Part model, mm, in its own coordinate system. Round coordinates to 2 decimals unless told otherwise and drop trailing zeros. Write each loop counter-clockwise with the first axis right and the second up, starting at its lowest first coordinate (ties: lowest second). Pieces come first, ordered by that corner, then holes.
1) Saw through at B-B on x = 0. Write the cut outline in (y, z), and give its area (3 significant figures).
2) Drill centre lines: L1, parallel to X at y = 1.85, z = 24.5; L2, parallel to X at y = 2.3, z = -8; L3, parallel to X at y = 1.8, z = -25.5. Where is each one in solid material? Low to high.
3) Saw through at A-A on z = 3.5. Write the cut outline in (x, y).
4) Saw through at C-C on y = 1.35. Count the separate pieces of the cut face and the enclosed holes in it, and give its area (3 significant figures).
5) Saw through at D-D on x = -42. Write the cut outline in (y, z).
6) Flat gauge pin, fed straight in: pin 1 (2.5 mm diameter, centred on x = -55, z = -24.5, fed in from +Y). Where does the tip first touch, or does it go through?
```python
from build123d import *

# Parameters (mm, degrees)
SKETCH_1_W          = 120
SKETCH_1_H          = 60
EXTRUDE_1_DEPTH     = 3
SKETCH_2_R          = 1.5
CUT_EXTRUDE_1_DEPTH = 68.149087857
SKETCH_3_R          = 1.5
CUT_EXTRUDE_2_DEPTH = 68.149087857
FILLET_1_R          = 5
SKETCH_4_W          = 30
SKETCH_4_H          = 40
CUT_EXTRUDE_3_DEPTH = 68.149087857
FILLET_2_R          = 5


with BuildPart() as part:
    # Sketch 1 → Extrude 1 (new body)
    with BuildSketch(Plane(origin=(0, 0, 0), x_dir=(1, 0, 0), z_dir=(0, 1, 0))):
        Rectangle(SKETCH_1_W, SKETCH_1_H)
    extrude(amount=EXTRUDE_1_DEPTH)

    # Sketch 2 → Cut-Extrude 1 (cut, through all)
    with BuildSketch(Plane(origin=(0, 3, 0), x_dir=(1, 0, 0), z_dir=(0, 1, 0))):
        with Locations(Location((-55, 24.5, 0), (0, 0, 270))):
            Circle(SKETCH_2_R)
        with Locations(Location((-15, 24.5, 0), (0, 0, 270))):
            Circle(SKETCH_2_R)
        with Locations(Location((-55, -24.5, 0), (0, 0, 90))):
            Circle(SKETCH_2_R)
        with Locations(Location((-15, -24.5, 0), (0, 0, 90))):
            Circle(SKETCH_2_R)
        with Locations(Location((15, -24.5, 0), (0, 0, 270))):
            Circle(SKETCH_2_R)
        with Locations(Location((55, -24.5, 0), (0, 0, 270))):
            Circle(SKETCH_2_R)
        with Locations(Location((15, 24.5, 0), (0, 0, 90))):
            Circle(SKETCH_2_R)
        with Locations(Location((55, 24.5, 0), (0, 0, 90))):
            Circle(SKETCH_2_R)
    extrude(amount=-CUT_EXTRUDE_1_DEPTH, mode=Mode.SUBTRACT)

    # Sketch 3 → Cut-Extrude 2 (cut, through all)
    with BuildSketch(Plane(origin=(0, 3, 0), x_dir=(1, 0, 0), z_dir=(0, 1, 0))):
        with Locations(Location((0, 15, 0), (0, 0, 270))):
            Circle(SKETCH_3_R)
        with Locations(Location((0, -15, 0), (0, 0, 90))):
            Circle(SKETCH_3_R)
    extrude(amount=-CUT_EXTRUDE_2_DEPTH, mode=Mode.SUBTRACT)

    # Fillet 1
    fillet_1_edges = [part.edges().sort_by_distance(p)[0] for p in [
        (60, 1.5, 30),
        (-60, 1.5, 30),
        (-60, 1.5, -30),
        (60, 1.5, -30),
    ]]
    fillet(fillet_1_edges, radius=FILLET_1_R)

    # Sketch 4 → Cut-Extrude 3 (cut, through all)
    with BuildSketch(Plane(origin=(0, 3, 0), x_dir=(1, 0, 0), z_dir=(0, 1, 0))):
        with Locations((35, 0)):
            Rectangle(SKETCH_4_W, SKETCH_4_H)
        with Locations((-35, 0)):
            Rectangle(SKETCH_4_W, SKETCH_4_H)
    extrude(amount=-CUT_EXTRUDE_3_DEPTH, mode=Mode.SUBTRACT)

    # Fillet 2
    fillet_2_edges = [part.edges().sort_by_distance(p)[0] for p in [
        (50, 1.5, -20),
        (50, 1.5, 20),
        (20, 1.5, 20),
        (20, 1.5, -20),
        (-20, 1.5, -20),
        (-20, 1.5, 20),
        (-50, 1.5, 20),
        (-50, 1.5, -20),
    ]]
    fillet(fillet_2_edges, radius=FILLET_2_R)


solid = part.part
```
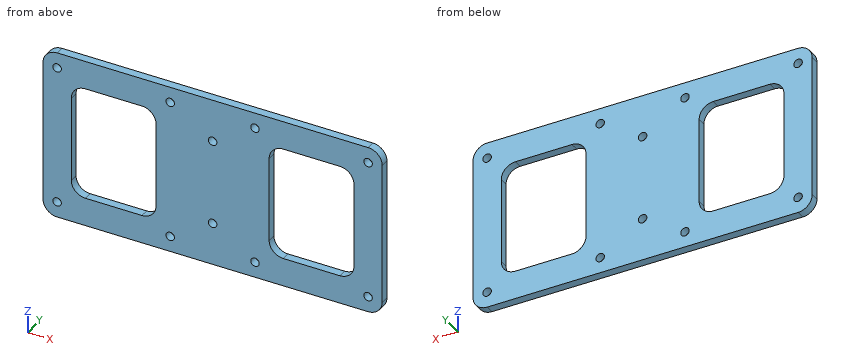
Completed:
1. outline: (0, -30) - (3, -30) - (3, -16.5) - (0, -16.5) - close; (0, -13.5) - (3, -13.5) - (3, 13.5) - (0, 13.5) - close; (0, 16.5) - (3, 16.5) - (3, 30) - (0, 30) - close
1. area: 162 mm2
2. L1: x = -60 to -56.5, -53.5 to -16.5, -13.5 to 13.5, 16.5 to 53.5, 56.5 to 60
2. L2: x = -60 to -50, -20 to 20, 50 to 60
2. L3: x = -59.97 to -56.12, -53.88 to -16.12, -13.88 to 13.88, 16.12 to 53.88, 56.12 to 59.97
3. outline: (-60, 0) - (-50, 0) - (-50, 3) - (-60, 3) - close; (-20, 0) - (20, 0) - (20, 3) - (-20, 3) - close; (50, 0) - (60, 0) - (60, 3) - (50, 3) - close
4. separate pieces: 1
4. enclosed holes: 12
4. area: 4,750 mm2
5. outline: (0, -30) - (3, -30) - (3, -20) - (0, -20) - close; (0, 20) - (3, 20) - (3, 30) - (0, 30) - close
6. pin 1: passes through
